Check sheet for the drawn part. Datum: minimum x, y, z corner. Units: mm. A direction names the side the tool comes from. Give positions to 0.01 mm unless a question says otherwise; leave off trailing zeros. Order: outer loops, then holes, each group sorted by start corner. A loop starts at its lowest first (then second) coordinate and runs counter-clockwise, first axis right, second up.
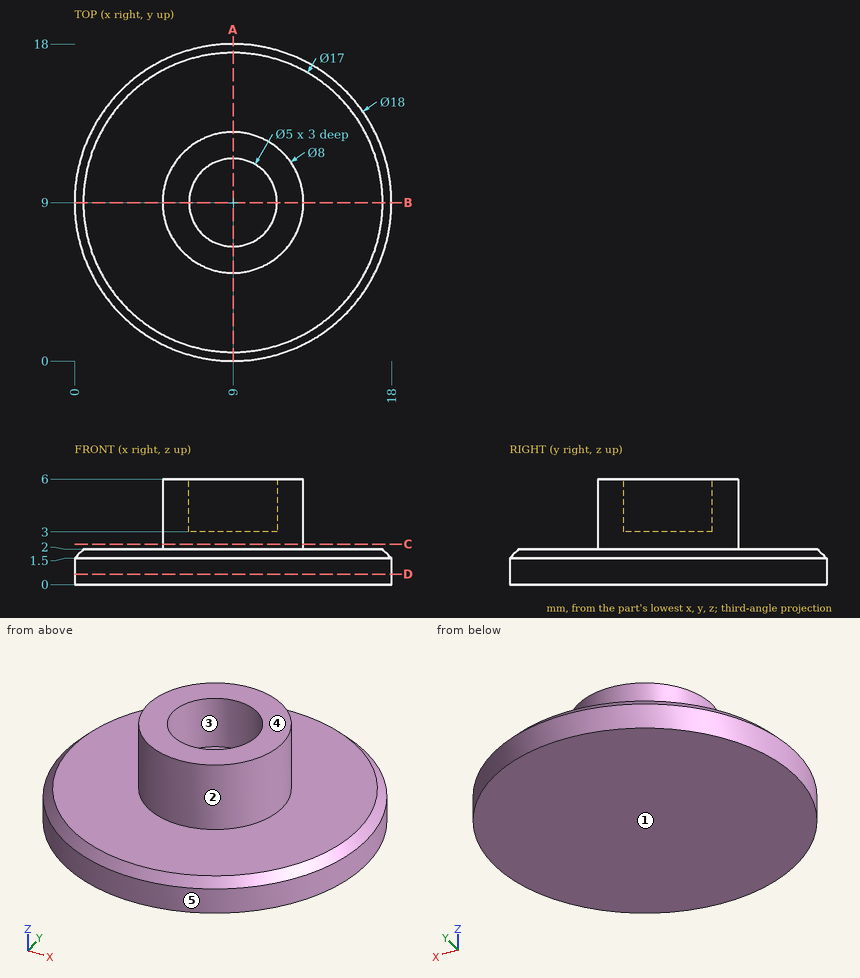
(1) Section check A-A, the plane x = 9. Enter the section's corners in (y, z).
Solved:
outline: (0, 0) - (18, 0) - (18, 1.5) - (17.5, 2) - (13, 2) - (13, 6) - (11.5, 6) - (11.5, 3) - (6.5, 3) - (6.5, 6) - (5, 6) - (5, 2) - (0.5, 2) - (0, 1.5) - close
(2) Go/stop test with a flat-tipped pin: pin 1 (10 mm diameter, centred on x = 8.5, y = 15.5, fed in from +Z). Record where the tip stops, or that it passes through.
Solved:
pin 1: stops at z = 6
(3) Release check for a two-part mould opening along X. For the marked faces 3, 4 and 5 record: pulls with the +X half, pulls with the -X half, needs draft (parallel to the pull), parting line crosses it, or undercut.
Solved:
face 3: undercut
face 4: needs draft
face 5: parting line crosses it
(4) Section check D-D, the plane z = 0.6. Enter the section's corners in (x, y).
Solved:
outline: circle Ø18 at (9, 9)
(5) Set-up check for the marked faces 1 and 2: record each of +Z, -Z, +X, -X, +Y, -Y from which the full face is reachable in a straight line by a thin tool's end or side.
Solved:
face 1: -Z, +X, -X, +Y, -Y
face 2: +Z
(6) Scan lines: line 1 (Y direction, x = 9, z = 3.9); line 2 (Z direction, x = 5, y = 6.5); line 3 (X direction, y = 10.5, z = 3.8). Record each from-to range of solid material in increasing order.
Solved:
line 1: y = 5 to 6.5, 11.5 to 13
line 2: z = 0 to 2
line 3: x = 5.29 to 7, 11 to 12.71
(7) Section check C-C, the plane z = 2.3. Enter the section's corners in (x, y).
Solved:
outline: circle Ø8 at (9, 9)
